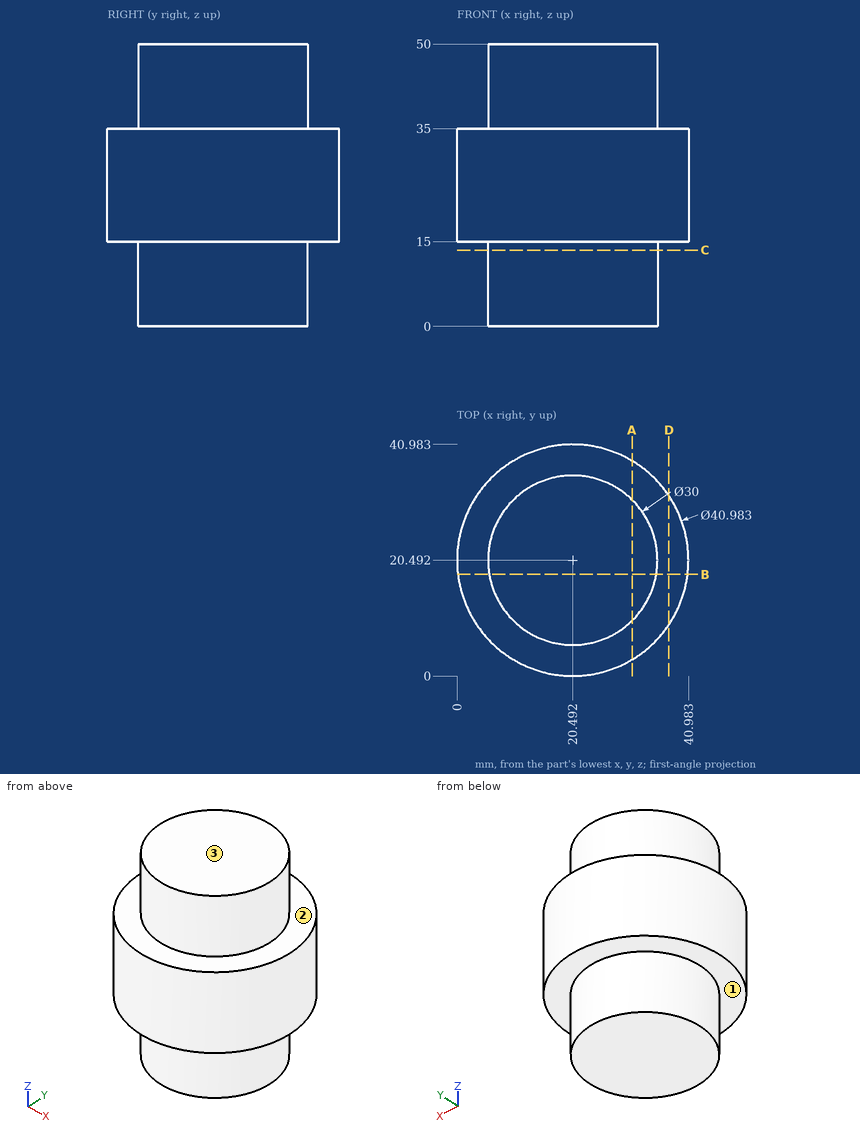
Verification items for this drawing (mm, ordinates from the low corner). A direction names the side the tool comes from. Coordinates: 2 decimals unless noted, no trailing zeros. Order: outer loops, then holes, each group sorted by start corner. A loop starts at its lowest first (then second) coordinate and runs counter-clockwise, first axis right, second up.
Q1. Sectioned sample at B-B on y = 18. Record the cut outline in (x, z).
Reply:
outline: (0.15, 15) - (5.7, 15) - (5.7, 0) - (35.28, 0) - (35.28, 15) - (40.83, 15) - (40.83, 35) - (35.28, 35) - (35.28, 50) - (5.7, 50) - (5.7, 35) - (0.15, 35) - close
Q2. Sectioned sample at D-D on x = 37.5. Record the cut outline in (y, z), and give its area (3 significant figures).
Reply:
outline: (9.06, 15) - (31.92, 15) - (31.92, 35) - (9.06, 35) - close
area: 457 mm2
Q3. Sectioned sample at C-C on z = 13.5. Record the cut outline in (x, y).
Reply:
outline: circle Ø30 at (20.49, 20.49)
Q4. Tool access check on the marked faces 1, 2 and 3. Record the directions out of +Z, -Z, +X, -X, +Y, -Y that give a thin tool (end or side, any length) a straight path to the whole face; none if there is none.
Reply:
face 1: -Z
face 2: +Z
face 3: +Z, +X, -X, +Y, -Y
Q5. Depth check by flat-ended pin: pin 1 Ø6 at (x, z) = (31, 6.5) entering from +Y; pin 2 Ø1.5 at (x, z) = (15, 10) entering from +Y; pin 3 Ø6 at (x, z) = (5, 26) entering from -Y. Enter the tip coordinate at first touch or a pass-through.
Reply:
pin 1: stops at y = 33.48
pin 2: stops at y = 34.72
pin 3: stops at y = 4.25
Q6. Sectioned sample at A-A on x = 31. Record the cut outline in (y, z) (1 decimal).
Reply:
outline: (2.9, 15) - (9.8, 15) - (9.8, 0) - (31.2, 0) - (31.2, 15) - (38.1, 15) - (38.1, 35) - (31.2, 35) - (31.2, 50) - (9.8, 50) - (9.8, 35) - (2.9, 35) - close
Q7. Thickness scan on probe 1 along Z at (x, y) = (31, 3); probe 2 along Y at (x, z) = (9, 28) (1 decimal); probe 3 along Y at (x, z) = (12, 40.5) (1 decimal). Record the ranges inside material, lowest first.
Reply:
probe 1: z = 15 to 35
probe 2: y = 3.5 to 37.5
probe 3: y = 8.1 to 32.9
